Part model, mm, in its own coordinate system. Face numbers are marked on the shaded views. Give positions to 0.01 mm unless a question says otherwise; leave off trailing zeros. Order: outer loops, then holes, each group sorted by start corner. A loop starts at its lowest first (then second) coordinate and runs counter-clockwise, first axis right, second up.
1. Slice it at C-C on y = 3. List the corners of the cut face in (x, z) (3 decimals).
2. Drop a flat-ended pin along its axis: pin 1 Ø0.6 at (x, y) = (0, -1.5) entering from +Z. Give the stop position or say it passes through.
3. Slice it at D-D on z = 0.4. List the corners of the cut face in (x, y) (3 decimals), and give its area (3 significant figures).
4. Slice it at A-A on y = -1. List the corners of the cut face in (x, z).
5. Probe line 1 (X direction, y = 1, z = 0.6) (3 decimals); line 2 (X direction, y = -2, z = 0.85); line 3 (Z direction, x = 0, y = 2.5) (3 decimals). List the from-to ranges inside material, lowest first.
6. Slice it at B-B on x = 1.45. List the corners of the cut face in (y, z) (3 decimals).
7. Mould opens along Z. For the marked faces 1, 2 and 3 say: +Z half, -Z half, draft (parallel to the pull), parting line (faces both ways), or undercut.
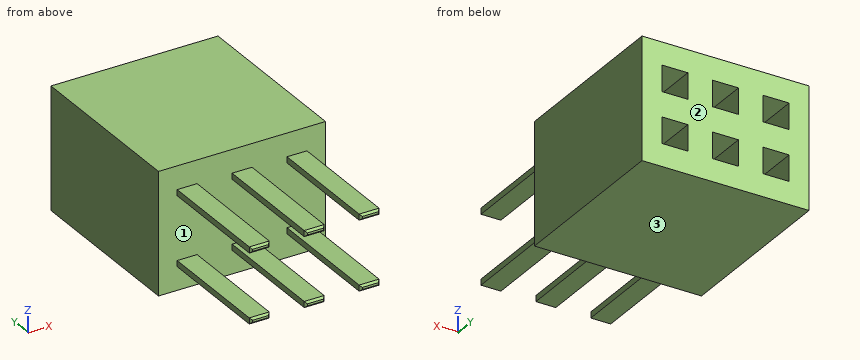
from build123d import *

# Parameters (mm, degrees)
ESQUISSE2_W             = 4.19
ESQUISSE2_H             = 3.05
BOSS_EXTRU_1_DEPTH      = 4.4
ESQUISSE4_W             = 0.65
ESQUISSE4_H             = 0.65
ENL_V_MAT_EXTRU_1_DEPTH = 3.5
ESQUISSE5_W             = 0.5
ESQUISSE5_H             = 0.15
BOSS_EXTRU_2_DEPTH      = 3
CHANFREIN1_SIZE         = 0.05


with BuildPart() as part:
    # Esquisse2 → Boss.-Extru.1 (new body)
    with BuildSketch(Plane(origin=(0, 0, 0), x_dir=(1, 0, 0), z_dir=(0, 1, 0))):
        Rectangle(ESQUISSE2_W, ESQUISSE2_H)
    extrude(amount=BOSS_EXTRU_1_DEPTH)

    # Esquisse4 → Enlèv. mat.-Extru.1 (cut)
    with BuildSketch(Plane(origin=(0, 4.4, 0), x_dir=(1, 0, 0), z_dir=(0, 1, 0))):
        with Locations((-1.27, 0.635)):
            Rectangle(ESQUISSE4_W, ESQUISSE4_H)
        with Locations((0, 0.635)):
            Rectangle(ESQUISSE4_W, ESQUISSE4_H)
        with Locations((1.27, 0.635)):
            Rectangle(ESQUISSE4_W, ESQUISSE4_H)
        with Locations((-1.27, -0.635)):
            Rectangle(ESQUISSE4_W, ESQUISSE4_H)
        with Locations((0, -0.635)):
            Rectangle(ESQUISSE4_W, ESQUISSE4_H)
        with Locations((1.27, -0.635)):
            Rectangle(ESQUISSE4_W, ESQUISSE4_H)
    extrude(amount=-ENL_V_MAT_EXTRU_1_DEPTH, mode=Mode.SUBTRACT)

    # Esquisse5 → Boss.-Extru.2 (add)
    with BuildSketch(Plane.XZ):
        with Locations((-1.377426973, 0.868741936)):
            Rectangle(ESQUISSE5_W, ESQUISSE5_H)
        with Locations((0, 0.868741936)):
            Rectangle(ESQUISSE5_W, ESQUISSE5_H)
        with Locations((1.377426973, 0.868741936)):
            Rectangle(ESQUISSE5_W, ESQUISSE5_H)
        with Locations((-1.377426973, -0.868741936)):
            Rectangle(ESQUISSE5_W, ESQUISSE5_H)
        with Locations((0, -0.868741936)):
            Rectangle(ESQUISSE5_W, ESQUISSE5_H)
        with Locations((1.377426973, -0.868741936)):
            Rectangle(ESQUISSE5_W, ESQUISSE5_H)
    extrude(amount=BOSS_EXTRU_2_DEPTH)

    # Chanfrein1
    chanfrein1_edges = [part.edges().sort_by_distance(p)[0] for p in [
        (0.25, -3, 0.868741936),
        (0, -3, 0.943741936),
        (-0.25, -3, 0.868741936),
        (0, -3, 0.793741936),
        (1.627426973, -3, 0.868741936),
        (1.377426973, -3, 0.943741936),
        (1.127426973, -3, 0.868741936),
        (1.377426973, -3, 0.793741936),
        (-1.127426973, -3, -0.868741936),
        (-1.377426973, -3, -0.793741936),
        (-1.627426973, -3, -0.868741936),
        (-1.377426973, -3, -0.943741936),
        (0.25, -3, -0.868741936),
        (0, -3, -0.793741936),
        (-0.25, -3, -0.868741936),
        (0, -3, -0.943741936),
        (1.627426973, -3, -0.868741936),
        (1.377426973, -3, -0.793741936),
        (1.127426973, -3, -0.868741936),
        (1.377426973, -3, -0.943741936),
        (-1.127426973, -3, 0.868741936),
        (-1.377426973, -3, 0.943741936),
        (-1.627426973, -3, 0.868741936),
        (-1.377426973, -3, 0.793741936),
    ]]
    chamfer(chanfrein1_edges, length=CHANFREIN1_SIZE)


solid = part.part
Data:
1. outline: (-2.095, -1.525) - (2.095, -1.525) - (2.095, 1.525) - (-2.095, 1.525) - close; hole (-1.595, -0.96) - (-0.945, -0.96) - (-0.945, -0.31) - (-1.595, -0.31) - close; hole (-1.595, 0.31) - (-0.945, 0.31) - (-0.945, 0.96) - (-1.595, 0.96) - close; hole (-0.325, -0.96) - (0.325, -0.96) - (0.325, -0.31) - (-0.325, -0.31) - close; hole (-0.325, 0.31) - (0.325, 0.31) - (0.325, 0.96) - (-0.325, 0.96) - close; hole (0.945, -0.96) - (1.595, -0.96) - (1.595, -0.31) - (0.945, -0.31) - close; hole (0.945, 0.31) - (1.595, 0.31) - (1.595, 0.96) - (0.945, 0.96) - close
2. pin 1: stops at z = 0.94
3. outline: (-2.095, 0) - (2.095, 0) - (2.095, 4.4) - (1.595, 4.4) - (1.595, 0.9) - (0.945, 0.9) - (0.945, 4.4) - (0.325, 4.4) - (0.325, 0.9) - (-0.325, 0.9) - (-0.325, 4.4) - (-0.945, 4.4) - (-0.945, 0.9) - (-1.595, 0.9) - (-1.595, 4.4) - (-2.095, 4.4) - close
3. area: 11.6 mm2
4. outline: (-1.63, -0.94) - (-1.13, -0.94) - (-1.13, -0.79) - (-1.63, -0.79) - close; (-1.63, 0.79) - (-1.13, 0.79) - (-1.13, 0.94) - (-1.63, 0.94) - close; (-0.25, -0.94) - (0.25, -0.94) - (0.25, -0.79) - (-0.25, -0.79) - close; (-0.25, 0.79) - (0.25, 0.79) - (0.25, 0.94) - (-0.25, 0.94) - close; (1.13, -0.94) - (1.63, -0.94) - (1.63, -0.79) - (1.13, -0.79) - close; (1.13, 0.79) - (1.63, 0.79) - (1.63, 0.94) - (1.13, 0.94) - close
5. line 1: x = -2.095 to -1.595, -0.945 to -0.325, 0.325 to 0.945, 1.595 to 2.095
5. line 2: x = -1.63 to -1.13, -0.25 to 0.25, 1.13 to 1.63
5. line 3: z = -1.525 to -0.96, -0.31 to 0.31, 0.96 to 1.525
6. outline: (-3, -0.894) - (-2.95, -0.944) - (0, -0.944) - (0, -1.525) - (4.4, -1.525) - (4.4, -0.96) - (0.9, -0.96) - (0.9, -0.31) - (4.4, -0.31) - (4.4, 0.31) - (0.9, 0.31) - (0.9, 0.96) - (4.4, 0.96) - (4.4, 1.525) - (0, 1.525) - (0, 0.944) - (-2.95, 0.944) - (-3, 0.894) - (-3, 0.844) - (-2.95, 0.794) - (0, 0.794) - (0, -0.794) - (-2.95, -0.794) - (-3, -0.844) - close
7. face 1: undercut
7. face 2: draft
7. face 3: -Z half
